```python
from build123d import *

# Parameters (mm, degrees)
PAD_DEPTH         = 20
SKETCH003_R       = 2
PAD001_DEPTH      = 7
POCKET001_DEPTH   = 20.001
SKETCH002_R       = 1.5
POCKET_DEPTH      = 13.001
POCKET_DEPTH_BACK = -13.001


with BuildPart() as part:
    # Binder → Pad (new body)
    with BuildSketch(Plane(origin=(0, 0, 0), x_dir=(0, 1, 0), z_dir=(0, 0, 1))):
        with BuildLine():
            ThreePointArc((12.857143, 4.116294), (0, 13.5), (-12.857143, 4.116294))
            ThreePointArc((-12.857143, 4.116294), (-12.964071, 3.664472), (-13, 3.201562))
            Line((-13, 3.201562), (-13, -3.201562))
            ThreePointArc((-13, -3.201562), (-12.964071, -3.664472), (-12.857143, -4.116294))
            ThreePointArc((-12.857143, -4.116294), (0, -13.5), (12.857143, -4.116294))
            ThreePointArc((12.857143, -4.116294), (12.964071, -3.664472), (13, -3.201562))
            Line((13, -3.201562), (13, 3.201562))
            ThreePointArc((13, 3.201562), (12.964071, 3.664472), (12.857143, 4.116294))
        make_face()
    extrude(amount=PAD_DEPTH)

    # Sketch003 (on Face3 of Pad) → Pad001 (join)
    with BuildSketch(Plane.XZ.offset(13)):
        with BuildLine():
            ThreePointArc((16, 0), (21, 5), (16, 10))
            Line((16, 10), (-16, 10))
            ThreePointArc((-16, 10), (-21, 5), (-16, 0))
            Line((16, 0), (-16, 0))
        make_face()
        with Locations((16, 5)):
            Circle(SKETCH003_R, mode=Mode.SUBTRACT)
        with Locations((-16, 5)):
            Circle(SKETCH003_R, mode=Mode.SUBTRACT)
    extrude(amount=-PAD001_DEPTH)

    # Sketch → Pocket001 (cut, through all)
    with BuildSketch(Plane.XY):
        with BuildLine():
            ThreePointArc((-3.201562, 10), (-10.5, 0), (-3.201562, -10))
            Line((-3.201562, -10), (3.201562, -10))
            ThreePointArc((3.201562, -10), (10.5, 0), (3.201562, 10))
            Line((-3.201562, 10), (3.201562, 10))
        make_face()
    extrude(amount=POCKET001_DEPTH, mode=Mode.SUBTRACT)

    # Sketch002 → Pocket (cut, two sides)
    with BuildSketch(Plane.XZ) as pocket_sk:
        with Locations((0, 5)):
            Circle(SKETCH002_R)
        with Locations((0, 15)):
            Circle(SKETCH002_R)
    extrude(amount=-POCKET_DEPTH, mode=Mode.SUBTRACT)
    extrude(pocket_sk.sketch, amount=-POCKET_DEPTH_BACK, mode=Mode.SUBTRACT)


solid = part.part
```
Part model, mm, in its own coordinate system. A direction names the side the tool comes from. Coordinates: 2 decimals unless noted, no trailing zeros. Order: outer loops, then holes, each group sorted by start corner. A loop starts at its lowest first (then second) coordinate and runs counter-clockwise, first axis right, second up. Notation, with made-up numbers: (80.25, 4) -> (86.25, 4) arc R36 cw to (86.25, 40) -> close; hole circle Ø6 at (-11, 87.25). An arc over 180 degrees is marked (long way). Put each result on its own line as item: value. Start each with the question number.
(1) Band-saw the part on C-C (y = 4.5). Give the cut face in (x, z), then the cut area to 3 significant figures.
(2) Band-saw the part on A-A (z = 5). Count the separate pieces of the cut face and the enclosed holes in it, then the cut area to 3 significant figures.
(3) Band-saw the part on B-B (z = 15). Give the cut face in (x, y), then the cut area to 3 significant figures.
(4) Probe line 1 along Z through (x, y) = (0, -11.25); line 2 along Z through (x, y) = (16, -10); line 3 along Y through (x, z) = (2, 3.5). List the from-to ranges inside material, lowest first. Write a range as [from, to].
(5) Which spindle directions (+Z, -Z, +X, -X, +Y, -Y) get a long thin tool onto all of the face, cutting with end or side? Do faces 4 (the face through (10.5, -0.2, 9.9)), 5 (the face through (-12, -10, 10)), 6 (the face through (16.5, -6, 7.3)), 7 (the face through (13, -10, 10)), 8 (the face through (-3.658, 12.965, 9.86)). Say none if no direction does.
(6) Band-saw the part on D-D (x = -8.5). Give the cut face in (y, z).
(7) Mould opens along X. For faces 1 (the face through (0, 13, 10)), 2 (the face through (-21, -10, 5)), 3 (the face through (0, 10, 10)) say: pulls with the +X half, pulls with the -X half, needs draft (parallel to the pull), parting line crosses it, or undercut.
(8) Pin check, flat tips, straight feed: pin 1 Ø5 at (y, z) = (-8.5, 7.5) entering from +X; pin 2 Ø2.5 at (x, z) = (0, 5) entering from -Y; pin 3 Ø3 at (y, z) = (3, 6.5) entering from +X; pin 4 Ø6 at (y, z) = (-4.5, 17) entering from -X. Stop position of each tip, or through.
Determined:
1. outline: (-12.73, 0) -> (-9.49, 0) -> (-9.49, 20) -> (-12.73, 20) -> close; (9.49, 0) -> (12.73, 0) -> (12.73, 20) -> (9.49, 20) -> close
1. area: 130 mm²
2. separate pieces: 4
2. enclosed holes: 0
2. area: 318 mm²
3. outline: (-4.12, -12.86) arc R3 ccw to (-3.2, -13) -> (-1.5, -13) -> (-1.5, -10) -> (-3.2, -10) arc R10.5 cw to (-3.2, 10) -> (-1.5, 10) -> (-1.5, 13) -> (-3.2, 13) arc R3 ccw to (-4.12, 12.86) arc R13.5 ccw to start; (1.5, -13) -> (3.2, -13) arc R3 ccw to (4.12, -12.86) arc R13.5 ccw to (4.12, 12.86) arc R3 ccw to (3.2, 13) -> (1.5, 13) -> (1.5, 10) -> (3.2, 10) arc R10.5 cw to (3.2, -10) -> (1.5, -10) -> close
3. area: 208 mm²
4. line 1: z = [0, 3.5], [6.5, 13.5], [16.5, 20]
4. line 2: z = [0, 3], [7, 10]
4. line 3: y = [-13, -10], [10, 13]
5. face 4: +Z, -Z
5. face 5: +Z, -X, -Y
5. face 6: +Z, -Z, +X
5. face 7: +Z, +X, -Y
5. face 8: +Z, -Z, -X, +Y
6. outline: (-13, 0) -> (-6.16, 0) -> (-6.16, 20) -> (-10.49, 20) -> (-10.49, 10) -> (-13, 10) -> close; (6.16, 0) -> (10.49, 0) -> (10.49, 20) -> (6.16, 20) -> close
7. face 1: needs draft
7. face 2: pulls with the -X half
7. face 3: undercut
8. pin 1: stops at x = 21
8. pin 2: passes through
8. pin 3: stops at x = 13.42
8. pin 4: stops at x = -13.42
